Here's how the part is built. I have some questions about the finished solid (model axes, mm). A direction names the side the tool comes from. Coordinates: 2 decimals unless noted, no trailing zeros. Loops run counter-clockwise (first coordinate to the right, second up) from the corner with the lowest first, then second, coordinate; pieces in that order, holes last.
Autodesk Inventor part; units mm, degrees
ref_plane "Work Plane1" through (30.1625, 0, 0) normal (0, 0, -1) x (1, 0, 0)
ref_plane "YZ Plane" through (0, 0, 0) normal (1, 0, 0) x (0, 1, 0)
ref_plane "XZ Plane" through (0, 0, 0) normal (0, 1, 0) x (-1, 0, 0)
sketch "Sketch1" plane through (0, 0, 0) normal (0, 0, 1) x (1, 0, 0)
  line L0 (-3.9, 0) -> (35, 0)
  line L1 (35, 0) -> (35, 3)
  line L2 (35, 3) -> (2, 3)
  line L3 (2, 3) -> (1.3864, 2.6932)
  line L4 (1.3864, 2.6932) -> (0, 2.6932)
  line L5 (0, 2.6932) -> (0, 5)
  line L6 (-11.68, 0) -> (42.78, 0)
  line L7 (0, -1) -> (0, 6)
  line L8 (-3.9, 0) -> (-3.9, 4.6588)
  line L9 (0, 5) -> (-3.9, 4.6588)
  line L10 (2, 3) -> (0, 3) construction
  dimension "d0" = 35
  dimension "d1" = 33
  dimension "d2" = 0.6136
  dimension "d3" = 3.9
  dimension "d4" = 6
  dimension "d5" = 5.3865
  dimension "d9" = 10
  dimension "d10" = 5
revolve "Body" add sketch "Sketch1" angle 360 about axis through (-3.9, 0, 0) along (1, 0, 0)
sketch "Sketch2" plane through (-3.9, 0, 0) normal (-1, 0, 0) x (0, 0, 1)
  circle A0 centre (0, 0) radius 5
  line L0 (0, 0) -> (0, 4.6588)
  line L1 (-5, 0.8) -> (5, 0.8)
  line L2 (5, 0.8) -> (5, -0.8)
  line L3 (5, -0.8) -> (-5, -0.8)
  line L4 (-5, -0.8) -> (-5, 0.8)
  line L5 (-5, 0) -> (5, 0) construction
  line L6 (0, 0.8) -> (0, -0.8) construction
  dimension "d11" = 1.6
  dimension "d12" = 10
fillet "Fillet1" radius 0.25 1 edges at (-3.9, -4.6588, 0)
extrude "Slot" cut sketch "Sketch2" against normal blind 1.6 contours A0 L3 L1 | L2 L3 A0 | A0 L1 L2 | A0 L4 L1 | L3 L4 A0
thread "Thread"
chamfer "Chamfer1" distance 0.6135 distance2 0.6136 1 edges at (35, -3, 0) measured on face at (35, 0.7485, -0.6631)
ref_plane "Work Plane1" through (30.1625, 0, 0) normal (0, 0, -1) x (1, 0, 0)
equation "\"d11\" = SBR"
equation "\"d12\" = KOD"
equation "\"d14\" = RR"
equation "\"d19\" = STI"
equation "\"d15\" = GEL"
equation "\"d17\" = -0.5 * SPD + 0.5 * GD"
equation "\"d0\" = NLG"
equation "\"d1\" = GEL"
equation "\"d3\" = KOH"
equation "\"d4\" = GD"
equation "\"d5\" = BDM"
equation "\"d9\" = KOD"
equation "\"d10\" = KEWI"
equation "\"GD\" = NND"
equation "\"NLG\" = 35"
equation "\"GEL\" = 33"
equation "\"KOD\" = 10"
equation "\"KOH\" = 3.9"
equation "\"GAL\" = 0.61345 * PTC"
equation "\"SPD\" = NND - 1.2269 * PTC"
equation "\"BDM\" = 5.3865"
equation "\"GUL\" = 0.61345 * PTC"
equation "\"RR\" = 0.25"
equation "\"SBR\" = 1.6"
equation "\"STI\" = 1.6"
equation "\"KEWI\" = 5deg"
equation "\"PTC\" = 1"
equation "\"THREADDIA\" = 6"
equation "\"TOA\" = 30deg"
equation "\"NND\" = 6"
equation "\"GD1\" = THREADDIA - 1.2269 * PTC"
properties part number "ISO 1207 - M6 x 35" material "Stainless Steel, 440C"
1. I need wall thicknesses on line 1 along Z through (x, y) = (9.5, 0); line 2 along X through (y, z) = (-1.75, 4); line 3 along X through (y, z) = (-0.25, 4.75). Which ranges of each line are inside material? Lowest first, please.
2. I want a section at C-C (x = 10). Please give me the cut outline in (y, z).
3. On a 3-axis mill with a long thin cutter (end or side, diameter ignored), from which of +Z, -Z, +X, -X, +Y, -Y can I reach the whole of each face in a straight line? I mean faces 1 (the flat face through (-3, -0.8, 0)), 2 (the flat face through (35, 0, 0)). Say none if no direction works.
4. I want a section at B-B (z = 0). Please give me the cut outline in (x, y).
5. For pin 1 (6 mm diameter, centred on x = 11.5, y = -3, fed in from +Z); pin 2 (1.8 mm diameter, centred on x = -3, z = 1, fed in from +Y); pin 3 (0.8 mm diameter, centred on y = 0, z = -0.5, fed in from -X), each with a flat end and sliding along its axis, tell me the tip position at first contact or that it passes through.
6. We'd pull the mould along X, two halves only. Please class faces 3 (the conical face through (-2.22, -1.04, -4.69)), 4 (the cylindrical face through (0.68, -2.69, -0.12)), 5 (the cylindrical face through (18, -3, 0)): +X half, -X half, draft (parallel to the pull), parting line (faces both ways), or undercut.
7. I want a section at A-A (y = 0). Please give me the cut outline in (x, z).
Response values:
1. line 1: z = -3 to 3
1. line 2: x = -3.9 to 0
1. line 3: x = -2.3 to 0
2. outline: circle Ø6 at (0, 0)
3. face 1: +Z, -Z, -X
3. face 2: +Z, -Z, +X, +Y, -Y
4. outline: (-3.9, -4.43) arc R0.25 ccw to (-3.67, -4.68) - (0, -5) - (0, -2.69) - (1.39, -2.69) - (2, -3) - (34.39, -3) - (35, -2.39) - (35, 2.39) - (34.39, 3) - (2, 3) - (1.39, 2.69) - (0, 2.69) - (0, 5) - (-3.67, 4.68) arc R0.25 ccw to (-3.9, 4.43) - (-3.9, 0.8) - (-2.3, 0.8) - (-2.3, -0.8) - (-3.9, -0.8) - close
5. pin 1: stops at z = 3
5. pin 2: stops at y = 4.78
5. pin 3: stops at x = -2.3
6. face 3: -X half
6. face 4: undercut
6. face 5: draft
7. outline: (-2.3, -4.8) - (0, -5) - (0, -2.69) - (1.39, -2.69) - (2, -3) - (34.39, -3) - (35, -2.39) - (35, 2.39) - (34.39, 3) - (2, 3) - (1.39, 2.69) - (0, 2.69) - (0, 5) - (-2.3, 4.8) - close
